Input: part model. Units: mm. Frame: model coordinates. A direction names the side the tool comes from. Coordinates: 2 decimals unless noted, no trailing zeros. Write each loop counter-clockwise with the first axis right and the second up, starting at its lowest first coordinate (ties: lowest second). Pieces come first, ordered by that corner, then holes. Notation, with made-up numbers: M -32.75,9 L -14.75,9 A9 cw -14.75,13 Z; hole C 2.5,-14 d8. An arc over 180 degrees is marked long. Answer as a JSON object with one key per item and string values. Group by question number.
from build123d import *

# Parameters (mm, degrees)
SALIENTE_EXTRUIR3_DEPTH = 1
SALIENTE_EXTRUIR4_DEPTH = 2
SALIENTE_EXTRUIR5_DEPTH = 40
SALIENTE_EXTRUIR6_DEPTH = 2


with BuildPart() as part:
    # Croquis3 → Saliente-Extruir3 (new body)
    with BuildSketch(Plane(origin=(0, 62.385327456, 0), x_dir=(1, 0, 0), z_dir=(0, 1, 0))):
        with BuildLine():
            Line((-8.035911824, 0.88857317), (-4.660164738, 0.738374056))
            ThreePointArc((-4.660164738, 0.738374056), (-3.491878014, -6.094633439), (3.225323709, -4.38171595))
            Line((3.225323709, -4.38171595), (4.917369229, -7.202342932))
            ThreePointArc((4.917369229, -7.202342932), (-5.114744648, -8.849076594), (-8.035911824, 0.88857317))
        make_face()
    extrude(amount=SALIENTE_EXTRUIR3_DEPTH)

    # Croquis4 → Saliente-Extruir4 (add)
    with BuildSketch(Plane(origin=(0, 63.385327456, 0), x_dir=(1, 0, 0), z_dir=(0, 1, 0))):
        with BuildLine():
            Line((4.917369229, -7.202342932), (4.642987805, -6.74495119))
            ThreePointArc((4.642987805, -6.74495119), (-4.860151229, -8.418565495), (-7.493817117, 0.864453429))
            Line((-7.493817117, 0.864453429), (-8.035911824, 0.88857317))
            ThreePointArc((-8.035911824, 0.88857317), (-5.114744648, -8.849076594), (4.917369229, -7.202342932))
        make_face()
    extrude(amount=SALIENTE_EXTRUIR4_DEPTH)

    # Croquis1 → Saliente-Extruir5 (add)
    with BuildSketch(Plane(origin=(0, 62.385327456, 0), x_dir=(1, 0, 0), z_dir=(0, 1, 0))):
        with BuildLine():
            Line((-4.660164738, 0.738374056), (-3.38107943, 2.399345645))
            ThreePointArc((-3.38107943, 2.399345645), (0.723456308, 0.1886696), (3.976176138, -3.151108223))
            Line((3.976176138, -3.151108223), (3.225323709, -4.38171595))
            ThreePointArc((3.225323709, -4.38171595), (-3.491878014, -6.094633439), (-4.660164738, 0.738374056))
        make_face()
        with BuildLine():
            Line((-3.867867022, 0.128239376), (-3.043523867, 1.19870008))
            ThreePointArc((-3.043523867, 1.19870008), (0.147575108, -0.629578738), (2.769944661, -3.208123684))
            Line((2.769944661, -3.208123684), (2.357240199, -3.884524638))
            ThreePointArc((2.357240199, -3.884524638), (-2.936970885, -5.262605721), (-3.867867022, 0.128239376))
        make_face(mode=Mode.SUBTRACT)
    extrude(amount=SALIENTE_EXTRUIR5_DEPTH)

    # Croquis8 → Saliente-Extruir6 (add)
    with BuildSketch(Plane.XZ.offset(-62.385327456)):
        with BuildLine():
            ThreePointArc((3.121797308, 35.939024727), (2.663211319, 38.370313658), (1.621742308, 40.614597347))
            Line((1.621742308, 40.614597347), (-7.903634902, 55.858387398))
            Line((-7.903634902, 55.858387398), (-46.320213658, 31.853044728))
            Line((-46.320213658, 31.853044728), (-36.913147682, 16.798592231))
            ThreePointArc((-36.913147682, 16.798592231), (-35.343131478, 14.869681606), (-33.345658311, 13.38787594))
            Line((-33.345658311, 13.38787594), (-8.035911824, -0.88857317))
            ThreePointArc((-8.035911824, -0.88857317), (-5.114744648, 8.849076594), (4.917369229, 7.202342932))
            Line((4.917369229, 7.202342932), (3.121797308, 35.939024727))
        make_face()
    extrude(amount=-SALIENTE_EXTRUIR6_DEPTH)


solid = part.part
Q1. Access query for faces 1 (the cylindrical face through (2.674, 63.371, 38.337)), 2 (the cylindrical face through (0.11, 82.11, 0.6)), 3 (the cylindrical face through (-4.73, 64.37, 8.5)). Directions: +Z, -Z, +X, -X, +Y, -Y. A direction counts if a zero-diameter tool reaches every point of the face in a straight line with its end or side. Return the directions, or none.
Q2. Section A-A, the plane y = 82.5. Return the cut outline in (x, z).
Q3. Pin query (flat end, axial travel): pin 1 Ø8.5 at (x, z) = (-0.92, 2.14) entering from +Y; pin 2 Ø6 at (x, z) = (-17.5, 37.5) entering from +Y. Return the tip coordinate at first contact, or that it passes through.
Q4. Section C-C, the plane x = -16. Return the cut outline in (y, z), and give its area (3 significant figures).
Q5. Draft query along X for faces 4 (the cylindrical face through (-2.86, 82.11, 5.31)), 5 (the flat face through (-15, 64.385, 28)), 6 (the flat face through (-41.68, 63.37, 24.43)), 7 (the flat face through (4.032, 63.371, 21.37)). Return one class per face: released by +X, released by -X, zero draft, split by the parting line, or undercut.
Q6. Section B-B, the plane z = 31. Return the cut outline in (x, y), and give its area (3 significant figures).
Q7. Line query: line 1 (Y direction, x = -12.5, z = 26); line 2 (X direction, y = 64, z = 29); line 3 (Z direction, x = -5, y = 71). Output: solid intervals per line, ascending. Write a range as from..to.
Filled in:
{
 "1": {"face 1": "+Z, +X, +Y, -Y", "face 2": "+Y, -Y", "face 3": "+Y"},
 "2": {"outline": "M -4.66,-0.74 L -3.38,-2.4 A15.37 ccw 3.98,3.15 L 3.23,4.38 A4.72 ccw long Z; hole M -3.87,-0.13 L -3.04,-1.2 A14.37 ccw 2.77,3.21 L 2.36,3.88 A3.72 ccw long Z"},
 "3": {"pin 1": "y = 102.39", "pin 2": "y = 64.39"},
 "4": {"outline": "M 62.39,3.6 L 64.39,3.6 L 64.39,50.8 L 62.39,50.8 Z", "area": "94.4 mm^2"},
 "5": {"face 4": "undercut", "face 5": "zero draft", "face 6": "released by -X", "face 7": "released by +X"},
 "6": {"outline": "M -45.79,62.39 L 3.43,62.39 L 3.43,64.39 L -45.79,64.39 Z", "area": "98.4 mm^2"},
 "7": {"line 1": "62.39..64.39", "line 2": "-44.54..3.56", "line 3": "-0.23..4.51"}
}
